Geometry: final body of the model. Coordinates: model frame, mm. A direction names the side the tool comes from. Give positions to 0.01 mm unless a question says otherwise; leave off trailing zeros. Write each loop counter-clockwise with the first axis right and the second up, starting at its lowest first coordinate (ties: lowest second). Pieces come first, ordered by that corner, then holes. Notation, with made-up numbers: M -36.5,32 L -14.5,32 A15 ccw -14.5,54 Z; hole C -1,27 d3. An arc over 180 degrees is marked long. Use a Markdown table: item, result. Add a question column.
1) Section B-B on y = 18. Return the cut outline in (x, z).
2) Set-up query: faces 1 (the cylindrical face through (-26.487, 22.395, 4.805)), 2 (the flat face through (0, 0, 0)), 3 (the cylindrical face through (0.9, -22.4, 6.2)). Return all of +Z, -Z, +X, -X, +Y, -Y with unobstructed straight access to the full face (end or side cutting, diameter ignored); none if empty.
3) Section A-A on y = -24. Return the cut outline in (x, z).
4) Line query: line 1 (X direction, y = -24, z = 7); line 2 (Z direction, x = 25, y = 25). Output: solid intervals per line, ascending.
5) Draft query along Y for faces 4 (the flat face through (0, 30, 5)), 5 (the cylindrical face through (-26.05, -27.34, 4.93)), 6 (the flat face through (0, 0, 10)). Return one class per face: +Y half, -Y half, draft (parallel to the pull), parting line (faces both ways), or undercut.
6) Section D-D on y = 26. Return the cut outline in (x, z).
7) Section C-C on x = -2.5. Return the cut outline in (y, z).
Autodesk Inventor part; units mm, degrees
ref_plane "YZ Plane" through (0, 0, 0) normal (1, 0, 0) x (0, 1, 0)
ref_plane "XZ Plane" through (0, 0, 0) normal (0, 1, 0) x (-1, 0, 0)
ref_plane "XY Plane" through (0, 0, 0) normal (0, 0, 1) x (1, 0, 0)
sketch "Skizze1" plane through (0, 0, 0) normal (0, 0, 1) x (1, 0, 0)
  line L0 (-35, -30) -> (35, -30)
  line L1 (35, -30) -> (35, 30)
  line L2 (35, 30) -> (-35, 30)
  line L3 (-35, 30) -> (-35, -30)
  line L4 (-35, -30) -> (35, 30) construction
  line L5 (35, -30) -> (-35, 30) construction
  point P0 (0, 0)
  dimension "Breite" = 70
  dimension "Länge" = 60
extrude "Extrusion1" add sketch "Skizze1" along normal blind 10
sketch "Skizze2" plane through (0, 0, 10) normal (0, 0, 1) x (1, 0, 0)
  line L0 (-35, -30) -> (35, -30)
  line L1 (0, -42) -> (0, 42)
  point P0 (0, 0)
  point P1 (-25, -24)
  point P2 (25, -24)
  point P3 (0, 18)
  dimension "Abstand_bohrung_unten" = 6
  dimension "Abstand_Bohrung_oben" = 48
hole "Bohrung1" at (25, -24, 10) at (-25, -24, 10) direction (0, 0, -1) diameter 7 end through all
hole "Bohrung2" at (0, 18, 10) direction (0, 0, -1) diameter 12 end through all
sketch "Skizze5" plane through (-35, 30, 0) normal (0, 1, 0) x (1, 0, 0)
  line L0 (70, -10) -> (0, -10)
  line L1 (0, 0) -> (0, -10)
  line L2 (70, 0) -> (70, -10)
  point P0 (35, 0)
  point P1 (60, -5)
  point P2 (10, -5)
  dimension "d36" = 5
  dimension "d37" = 50
  dimension "d38" = 10
  dimension "d39" = 10
hole "Bohrung5" at (25, 30, 5) at (-25, 30, 5) direction (0, -1, 0) diameter 3 depth 15 tip angle 118
sketch "Skizze6" plane through (-35, -30, 0) normal (0, -1, 0) x (1, 0, 0)
  line L0 (0, 10) -> (70, 10)
  line L1 (70, 0) -> (70, 10)
  point P0 (35, 0)
  point P1 (35, 5)
  dimension "d47" = 5
  dimension "d48" = 35
hole "Bohrung6" at (0, -30, 5) direction (0, 1, 0) diameter 3 depth 15 tip angle 118
properties part number "ABI_Grundplatte"
Found:
| question | item | result |
|---|---|---|
| 1 | outline | M -35,0 L -6,0 L -6,10 L -35,10 Z; M 6,0 L 35,0 L 35,10 L 6,10 Z; hole C -25,5 d3; hole C 25,5 d3 |
| 2 | face 1 | +Y |
| 2 | face 2 | -Z, +X, -X, +Y, -Y |
| 2 | face 3 | -Y |
| 3 | outline | M -35,0 L -28.5,0 L -28.5,10 L -35,10 Z; M -21.5,0 L 21.5,0 L 21.5,10 L -21.5,10 Z; M 28.5,0 L 35,0 L 35,10 L 28.5,10 Z; hole C 0,5 d3 |
| 4 | line 1 | -35 to -28.5, -21.5 to 21.5, 28.5 to 35 |
| 4 | line 2 | 0 to 3.5, 6.5 to 10 |
| 5 | face 4 | +Y half |
| 5 | face 5 | undercut |
| 5 | face 6 | draft |
| 6 | outline | M -35,0 L 35,0 L 35,10 L -35,10 Z; hole C -25,5 d3; hole C 25,5 d3 |
| 7 | outline | M -30,0 L 12.55,0 L 12.55,10 L -30,10 Z; M 23.45,0 L 30,0 L 30,10 L 23.45,10 Z |
